Autodesk Inventor part; units mm, degrees
ref_plane "YZ Plane" through (0, 0, 0) normal (1, 0, 0) x (0, 1, 0)
ref_plane "XZ Plane" through (0, 0, 0) normal (0, 1, 0) x (-1, 0, 0)
ref_plane "XY Plane" through (0, 0, 0) normal (0, 0, 1) x (1, 0, 0)
sketch "Sketch1" plane through (0, 0, 0) normal (0, 1, 0) x (-1, 0, 0)
  line L0 (25.0064, 9.2593) -> (-5.9936, 9.2593)
  line L1 (-5.9936, 9.2593) -> (-5.9936, -3.7407)
  line L2 (-5.9936, -3.7407) -> (25.0064, -3.7407)
  line L3 (25.0064, -3.7407) -> (25.0064, 9.2593)
  point P0 (0, 0)
  dimension "d0" = 31
  dimension "d1" = 13
extrude "Extrusion1" add sketch "Sketch1" along normal blind 1.6
sketch "Sketch2" plane through (0, 1.6, 0) normal (0, 1, 0) x (1, 0, 0)
  line L0 (5.9936, -9.2593) -> (5.9936, 3.7407)
  line L1 (5.9936, 3.7407) -> (-25.0064, 3.7407)
  line L2 (5.3936, -6.4593) -> (5.3936, 1.1407)
  line L3 (5.3936, 1.1407) -> (2.7936, 1.1407)
  line L4 (2.7936, 1.1407) -> (2.7936, -6.4593)
  line L5 (2.7936, -6.4593) -> (5.3936, -6.4593)
  point P0 (0, 0)
  point P1 (5.9936, 1.1407)
  point P2 (5.9936, -6.4593)
  dimension "d9" = 2.6
  dimension "d10" = 7.6
  dimension "d12" = 2.6
  dimension "d13" = 0.6
extrude "Extrusion2" add sketch "Sketch2" along normal blind 2.8
sketch "Sketch3" plane through (0, 4.4, 0) normal (0, 1, 0) x (1, 0, 0)
  circle A0 centre (4.0936, -5.2593) radius 0.3
  circle A1 centre (4.0936, -2.6593) radius 0.3
  circle A2 centre (4.0936, -0.0593) radius 0.3
  line L0 (5.3936, -6.4593) -> (5.3936, 1.1407)
  line L1 (2.7936, -6.4593) -> (5.3936, -6.4593)
  point P0 (0, 0)
  dimension "d14" = 0.6
  dimension "d15" = 0.6
  dimension "d16" = 0.6
  dimension "d17" = 1.3
  dimension "d18" = 1.3
  dimension "d19" = 1.3
  dimension "d20" = 2
  dimension "d21" = 2
  dimension "d22" = 1.2
extrude "Extrusion3" add sketch "Sketch3" along normal blind 5.8
sketch "Sketch4" plane through (0, 1.6, 0) normal (0, 1, 0) x (1, 0, 0)
  line L0 (-24.1064, -7.6593) -> (-16.7064, -7.6593)
  line L1 (-16.7064, -7.6593) -> (-16.7064, 2.3407)
  line L2 (-16.7064, 2.3407) -> (-24.1064, 2.3407)
  line L3 (-24.1064, 2.3407) -> (-24.1064, -7.6593)
  line L4 (-25.0064, 3.7407) -> (-25.0064, -9.2593)
  line L5 (-25.0064, -9.2593) -> (5.9936, -9.2593)
  point P0 (0, 0)
  dimension "d25" = 7.4
  dimension "d26" = 10
  dimension "d27" = 0.9
  dimension "d28" = 1.6
extrude "Extrusion4" add sketch "Sketch4" along normal blind 5.6
sketch "Sketch5" plane through (0, 7.2, 0) normal (0, 1, 0) x (1, 0, 0)
  line L0 (-23.7064, -7.6593) -> (-18.7064, -7.6593)
  line L1 (-18.7064, -7.6593) -> (-18.7064, 2.3407)
  line L2 (-18.7064, 2.3407) -> (-23.7064, 2.3407)
  line L3 (-23.7064, 2.3407) -> (-23.7064, -7.6593)
  line L4 (-24.1064, -7.6593) -> (-16.7064, -7.6593)
  line L5 (-24.1064, 2.3407) -> (-16.7064, 2.3407)
  line L6 (-16.7064, -7.6593) -> (-16.7064, 2.3407)
  point P0 (0, 0)
  dimension "d31" = 5
  dimension "d32" = 0
  dimension "d33" = 0
  dimension "d34" = 2
extrude "Extrusion5" add sketch "Sketch5" along normal blind 3.4 contours L3 L2 L1 L0
ref_plane "Work Plane1" through (-24.1064, 7.2, -2.3407) normal (-0.9932, 0.1168, 0) x (0, 0, 1)
sketch "Sketch6" plane through (-24.1064, 7.2, -2.3407) normal (-0.9932, 0.1168, 0) x (0, 0, 1)
  line L0 (0, 3.4234) -> (0, 0)
  line L1 (0, 0) -> (10, 0)
  line L2 (0, 0) -> (10, 0)
  line L3 (10, 0) -> (10, 3.4234)
  line L4 (10, 3.4234) -> (0, 3.4234)
  line L5 (0, 3.4234) -> (10, 3.4234)
  point P0 (2.3407, -4.3341)
extrude "Extrusion6" add sketch "Sketch6" against normal blind 1
ref_plane "Work Plane2" through (-18.7064, 10.6, 7.6593) normal (-0.8619, -0.507, 0) x (0, 0, -1)
sketch "Sketch7" plane through (-18.7064, 10.6, 7.6593) normal (-0.8619, -0.507, 0) x (0, 0, -1)
  line L0 (0, 0) -> (0, 3.9446)
  line L1 (0, 3.9446) -> (10, 3.9446)
  line L2 (0, 3.9446) -> (10, 3.9446)
  line L3 (10, 3.9446) -> (10, 0)
  line L4 (10, 0) -> (0, 0)
  point P0 (7.6593, 18.621)
extrude "Extrusion7" add sketch "Sketch7" along normal blind 2
sketch "Sketch8" plane through (0, 10.6, 0) normal (0, 1, 0) x (1, 0, 0)
  circle A0 centre (-21.0064, -0.1593) radius 1.7
  circle A1 centre (-21.0064, -5.1593) radius 1.7
  line L0 (-18.7064, 2.3407) -> (-23.7064, 2.3407)
  line L1 (-23.7064, 2.3407) -> (-23.7064, -7.6593)
  point P0 (0, 0)
  dimension "d41" = 3.4
  dimension "d42" = 3.4
  dimension "d43" = 2.5
  dimension "d44" = 5
  dimension "d45" = 2.7
  dimension "d46" = 2.7
extrude "Extrusion8" cut sketch "Sketch8" against normal blind 2
sketch "Sketch9" plane through (0, 1.6, 0) normal (0, 1, 0) x (1, 0, 0)
  line L0 (-14.7064, -5.2593) -> (-10.7064, -5.2593)
  line L1 (-10.7064, -5.2593) -> (-10.7064, -0.2593)
  line L2 (-10.7064, -0.2593) -> (-14.7064, -0.2593)
  line L3 (-14.7064, -0.2593) -> (-14.7064, -5.2593)
  line L4 (-16.7064, -7.6593) -> (-16.7064, 2.3407)
  line L5 (5.9936, 3.7407) -> (-25.0064, 3.7407)
  point P0 (0, 0)
  dimension "d49" = 4
  dimension "d50" = 5
  dimension "d51" = 2
  dimension "d52" = 4
extrude "Extrusion9" add sketch "Sketch9" along normal blind 1.4
fillet "Fillet1" radius 0.2 4 edges at (-10.7064, 3, 2.7593) (-12.7064, 3, 5.2593) (-14.7064, 3, 2.7593) (-12.7064, 3, 0.2593)
equation "\"d18\" = d17"
equation "\"d19\" = d17"
equation "\"d46\" = d45"
properties part number "ACS712(prudovy snimac)"
Geometry check sheet. Reference: the model listing, model coordinates, mm. A direction names the side the tool comes from. Give positions to 0.01 mm unless a question says otherwise; leave off trailing zeros. Order: outer loops, then holes, each group sorted by start corner. A loop starts at its lowest first (then second) coordinate and runs counter-clockwise, first axis right, second up. Notation, with made-up numbers: (9.5, 52.25) - (39.5, 52.25) arc R18 ccw to (39.5, 73.25) - close; hole circle Ø4 at (-36, -35.75). An arc over 180 degrees is marked (long way). Answer in a Markdown table with one row per item. Add a question column.
Q1. Gauge pin test, flat ends, axial feed: pin 1 (3 mm diameter, centred on x = -8, z = -0.5, fed in from +Y); pin 2 (1 mm diameter, centred on y = 2.5, z = 3.5, fed in from +X); pin 3 (0.8 mm diameter, centred on x = 4, y = 3.5, fed in from -Z). Record the tip position at first contact, or that the pin passes through.
Q2. Mould release check, pull along X, two halves, no side actions. Record for faces 5 (the flat face through (-13, 3, 3)), 6 (the flat face through (-23.904, 8.924, 2.589)), 7 (the flat face through (5.994, 1, 3)): pulls with the +X half, pulls with the -X half, needs draft (parallel to the pull), parting line crosses it, or undercut.
Q3. Cross-section at B-B, the plane y = 5.25. Enter the section's corners in (x, z), then the cut area to 3 significant figures.
Q4. Tool access check on faces 1 (the flat face through (-24.106, 4, 3)), 2 (the flat face through (-21, 8.6, 5)), 3 (the flat face through (-20, 6, -2.341)), 4 (the flat face through (2.794, 3, 3)). Record the directions out of +Z, -Z, +X, -X, +Y, -Y that give a thin tool (end or side, any length) a straight path to the whole face; none if there is none.
Q5. Cross-section at C-C, the plane x = -12. Enter the section's corners in (y, z).
Q6. Cross-section at A-A, the plane y = 3.5. Enter the section's corners in (x, z).
Q7. Material ranges on probe 1 along X at (y, z) = (2.5, 3.25); probe 2 along X at (y, z) = (3, -0.5); probe 3 along X at (y, z) = (6.75, 1.75), recorded low to high. Write a range as from..to.
Check values:
| question | item | result |
|---|---|---|
| 1 | pin 1 | stops at y = 1.6 |
| 1 | pin 2 | stops at x = 5.39 |
| 1 | pin 3 | stops at z = -1.14 |
| 2 | face 5 | undercut |
| 2 | face 6 | pulls with the -X half |
| 2 | face 7 | pulls with the +X half |
| 3 | outline | (-24.11, -2.34) - (-16.71, -2.34) - (-16.71, 7.66) - (-24.11, 7.66) - close; circle Ø0.6 at (4.09, 0.06); circle Ø0.6 at (4.09, 2.66); circle Ø0.6 at (4.09, 5.26) |
| 3 | area | 74.8 mm^2 |
| 4 | face 1 | +Z, -Z, -X, +Y |
| 4 | face 2 | +Y |
| 4 | face 3 | -Z, +X, -X, +Y |
| 4 | face 4 | +Z, -Z, +Y |
| 5 | outline | (0, -3.74) - (1.6, -3.74) - (1.6, 0.26) - (2.8, 0.26) arc R0.2 ccw to (3, 0.46) - (3, 5.06) arc R0.2 ccw to (2.8, 5.26) - (1.6, 5.26) - (1.6, 9.26) - (0, 9.26) - close |
| 6 | outline | (-24.11, -2.34) - (-16.71, -2.34) - (-16.71, 7.66) - (-24.11, 7.66) - close; (2.79, -1.14) - (5.39, -1.14) - (5.39, 6.46) - (2.79, 6.46) - close |
| 7 | probe 1 | x = -24.11..-16.71, -14.71..-10.71, 2.79..5.39 |
| 7 | probe 2 | x = -24.11..-16.71, 2.79..5.39 |
| 7 | probe 3 | x = -24.11..-16.71 |
